Drawing for the job (mm, zero at the part's lowest x, y, z). A direction names the side the tool comes from. Round coordinates to 2 decimals unless told otherwise and drop trailing zeros. Loops run counter-clockwise (first coordinate to the right, second up) from the corner with the lowest first, then second, coordinate; pieces in that order, holes last. Notation, with made-up numbers: M 56,68.5 L 105,68.5 A31 ccw 105,100.5 Z; hole C 39.5,32 d10. An arc over 180 degrees is marked long. Use a Markdown table: item, result. Add a question column.
Q1. Cut at C-C (y = 34). Give the cut face in (x, z) (3 decimals).
Q2. Tool access for the marked faces 1, 2 and 3: list every direction of +Z, -Z, +X, -X, +Y, -Y with a clear straight run to the whole face (end or side of a thin tool).
Q3. Cut at A-A (z = 13.97). Give the cut face in (x, y).
Q4. Cut at D-D (x = 48.5). Give the cut face in (y, z).
Q5. Pin check, flat tips, straight feed: pin 1 (7.5 mm diameter, centred on y = 29.972, z = 13.97, fed in from +X); pin 2 (3 mm diameter, centred on x = 68, z = 3, fed in from -Y); pin 3 (7.5 mm diameter, centred on x = 8.2, y = 8.13, fed in from -Z) (3 decimals); pin 4 (12 mm diameter, centred on x = 71.5, y = 30.5, fed in from +Z). Stop position of each tip, or through.
Q6. Probe line 1 (Y direction, x = 20.05, z = 13.97); line 2 (Z direction, x = 31, y = 25); line 3 (X direction, y = 26.5, z = 6.25). List the from-to ranges inside material, lowest first. Write a range as from..to.
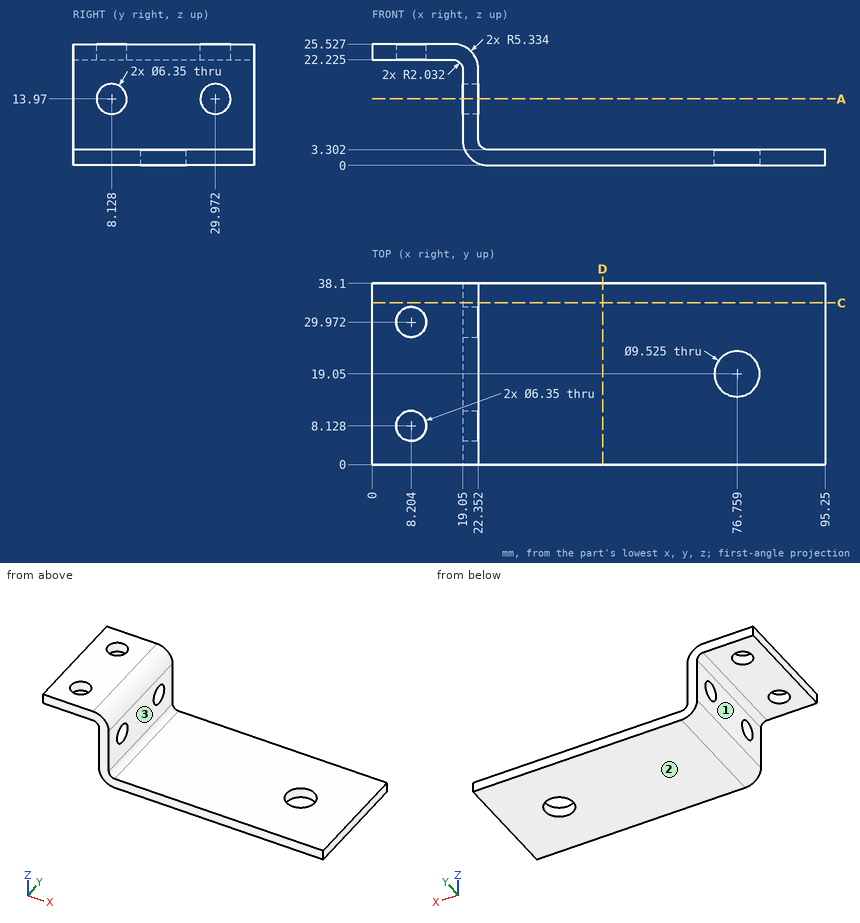
Checked values:
| question | item | result |
|---|---|---|
| 1 | outline | M 0,22.225 L 17.018,22.225 A2.032 cw 19.05,20.193 L 19.05,5.334 A5.334 ccw 24.384,0 L 95.25,0 L 95.25,3.302 L 24.384,3.302 A2.032 cw 22.352,5.334 L 22.352,20.193 A5.334 ccw 17.018,25.527 L 0,25.527 Z |
| 2 | face 1 | -Z, -X, +Y, -Y |
| 2 | face 2 | -Z, +X, -X, +Y, -Y |
| 2 | face 3 | +Z, +X, +Y, -Y |
| 3 | outline | M 19.05,0 L 22.35,0 L 22.35,4.95 L 19.05,4.95 Z; M 19.05,11.3 L 22.35,11.3 L 22.35,26.8 L 19.05,26.8 Z; M 19.05,33.15 L 22.35,33.15 L 22.35,38.1 L 19.05,38.1 Z |
| 4 | outline | M 0,0 L 38.1,0 L 38.1,3.3 L 0,3.3 Z |
| 5 | pin 1 | stops at x = 22.35 |
| 5 | pin 2 | stops at y = 0 |
| 5 | pin 3 | stops at z = 22.225 |
| 5 | pin 4 | stops at z = 3.3 |
| 6 | line 1 | y = 0..4.95, 11.3..26.8, 33.15..38.1 |
| 6 | line 2 | z = 0..3.3 |
| 6 | line 3 | x = 19.05..22.35 |
